Read the model definition and answer for the solid it produces. Units are mm, in the model's axes. A direction names the side the tool comes from. Give positions to 0.01 mm unless a question says otherwise; leave off trailing zeros. Write each loop counter-clockwise with the first axis right and the second up, starting at its lowest first coordinate (ties: lowest second). Pieces come first, ordered by that corner, then holes. Notation, with made-up numbers: M 59.5,-14.75 L 100.5,-14.75 A26 cw 100.5,23.25 Z; hole C 89,-11.5 d11. An arc over 180 degrees is marked long. Answer as CSV lines item,"result". Start each with the question number.
Solid Edge part; units mm, degrees
sketch "Sketch1" plane through (0, 0, 0) normal (-1, 0, 0) x (0, -1, 0)
  circle A0 centre (0, 0) radius 1.5
extrude "Protrusion1" add sketch "Sketch1" against normal blind 4
sketch "Sketch2" plane through (0, 0, 0) normal (-1, 0, 0) x (0, -1, 0)
  line L0 (-1.0355, -2.5) -> (1.0355, -2.5)
  line L1 (1.0355, -2.5) -> (2.5, -1.0355)
  line L2 (2.5, -1.0355) -> (2.5, 1.0355)
  line L3 (2.5, 1.0355) -> (1.0355, 2.5)
  line L4 (1.0355, 2.5) -> (-1.0355, 2.5)
  line L5 (-1.0355, 2.5) -> (-2.5, 1.0355)
  line L6 (-2.5, 1.0355) -> (-2.5, -1.0355)
  line L7 (-2.5, -1.0355) -> (-1.0355, -2.5)
extrude "Protrusion2" add sketch "Sketch2" along normal blind 5
sketch "Sketch3" plane through (-5, 0, 0) normal (-1, 0, 0) x (0, -1, 0)
  circle A0 centre (0, 0) radius 1.5
extrude "ExtrudedCutout_32" cut sketch "Sketch3" against normal blind 4
1. Find the intervals of material crossed by line 1 (Z direction, x = -2.5, y = 0); line 2 (X direction, y = 0.45, z = 1.2); line 3 (X direction, y = 1.35, z = 1.25), in increasing order. Write a range as [from, to].
2. Find section A-A on x = -2.5. Determine the outline of the cut face in (y, z).
3. Determine the mould class of faces 1 (the face through (-1, 0, 0)), 2 (the face through (-3.03, 1.5, 0.07)), 3 (the face through (-2.465, -1.757, -1.778)), 4 (the face through (-5, -2, 0)) for opening direction Z: +Z half, -Z half, draft (parallel to the pull), parting line (faces both ways), or undercut.
4. Find section D-D on x = -0.5. Determine the outline of the cut face in (y, z).
5. Given pin 1 (3 mm diameter, centred on x = 2, z = 0.5, fed in from -Y), flat-ended and moving along its own axis, determine where the tip first touches the part or whether it passes through.
6. For faces 5 (the face through (1.97, 1.5, 0.07)), 6 (the face through (4, 0, 0)), determine the directions among +Z, -Z, +X, -X, +Y, -Y from which every point of the face is accessible in a straight line to the end or side of a thin tool.
7. Find section B-B on z = 0. Determine the outline of the cut face in (x, y).
Computed:
1,line 1,"z = [-2.5, -1.5], [1.5, 2.5]"
1,line 2,"x = [-1, 4]"
1,line 3,"x = [-5, 0]"
2,outline,"M -2.5,-1.04 L -1.04,-2.5 L 1.04,-2.5 L 2.5,-1.04 L 2.5,1.04 L 1.04,2.5 L -1.04,2.5 L -2.5,1.04 Z; hole C 0,0 d3"
3,face 1,"undercut"
3,face 2,"undercut"
3,face 3,"-Z half"
3,face 4,"draft"
4,outline,"M -2.5,-1.04 L -1.04,-2.5 L 1.04,-2.5 L 2.5,-1.04 L 2.5,1.04 L 1.04,2.5 L -1.04,2.5 L -2.5,1.04 Z"
5,pin 1,"stops at y = -1.5"
6,face 5,"+X"
6,face 6,"+Z, -Z, +X, +Y, -Y"
7,outline,"M -5,-2.5 L 0,-2.5 L 0,-1.5 L 4,-1.5 L 4,1.5 L 0,1.5 L 0,2.5 L -5,2.5 L -5,1.5 L -1,1.5 L -1,-1.5 L -5,-1.5 Z"
